The model under review builds one solid part; all positions refer to its coordinate system, in mm. Round coordinates to 2 decimals unless told otherwise and drop trailing zeros. Write each loop counter-clockwise with the first axis right and the second up, starting at its lowest first coordinate (ties: lowest second). Pieces come first, ordered by that corner, then holes.
Item 1: Add section C-C (z = -26). Give the boundary of the cut face in (x, y) (3 decimals).
Item 2: Add section A-A (x = 9). Give the boundary of the cut face in (y, z) (3 decimals), plus the area to 3 significant figures.
Item 3: Add section D-D (y = 1.1). State how many separate pieces and enclosed holes the cut face has, plus the area to 3 significant figures.
Item 4: Draft analysis for pull direction X (two halves, no side actions). For faces 1 (the face through (13, 2, -1.384)), 2 (the face through (29, 2, -33.274)), state which applies: +X half, -X half, draft (parallel to the pull), parting line (faces both ways), or undercut.
Item 5: Add section B-B (z = -31). Give the boundary of the cut face in (x, y) (3 decimals).
Item 6: Clearance check with flat-ended pins moving along their axes: pin 1 Ø1.5 at (y, z) = (2.5, -21) entering from -X; pin 2 Ø1 at (y, z) = (1, -4) entering from +X; pin 3 Ø4.5 at (x, z) = (52.57, -11.63) entering from -Y. State where each tip first meets the part, or that it passes through.
Item 7: To check wall thickness, follow L1, parallel to Z at x = 14, y = 1.3 (3 decimals); L2, parallel to X at y = 1.3, z = -11.5; L3, parallel to Z at x = 4, y = 1. State the ranges of each line that lie inside material, in increasing order.
```python
from build123d import *

# Parameters (mm, degrees)
BOSS_EXTRUDE1_DEPTH   = 3.175
F_6_32_TAPPED_HOLE1_D = 2.7051
CUT_EXTRUDE1_REACH    = 69.902


with BuildPart() as part:
    # Sketch1 → Boss-Extrude1 (new body)
    with BuildSketch(Plane(origin=(0, 0, 0), x_dir=(1, 0, 0), z_dir=(0, 1, 0))):
        with BuildLine():
            Line((3.175, 0), (53.721, 0))
            ThreePointArc((53.721, 0), (55.96606403, 0.92993597), (56.896, 3.175))
            Line((56.896, 3.175), (56.896, 11.684))
            ThreePointArc((56.896, 11.684), (59.1058, 16.637), (56.896, 21.59))
            Line((56.896, 21.59), (56.896, 30.099))
            ThreePointArc((56.896, 30.099), (55.96606403, 32.34406403), (53.721, 33.274))
            Line((53.721, 33.274), (3.175, 33.274))
            ThreePointArc((3.175, 33.274), (0.92993597, 32.34406403), (0, 30.099))
            Line((0, 30.099), (0, 21.59))
            ThreePointArc((0, 21.59), (-2.2098, 16.637), (0, 11.684))
            Line((0, 11.684), (0, 3.175))
            ThreePointArc((0, 3.175), (0.92993597, 0.92993597), (3.175, 0))
        make_face()
        with BuildLine():
            Line((49.276, 26.797), (7.62, 26.797))
            ThreePointArc((7.62, 26.797), (5.23875, 24.41575), (7.62, 22.0345))
            Line((7.62, 22.0345), (7.62, 19.01825))
            Line((7.62, 19.01825), (4.445875862, 19.01825))
            ThreePointArc((4.445875862, 19.01825), (2.064625862, 16.637), (4.445875862, 14.25575))
            Line((4.445875862, 14.25575), (7.62, 14.25575))
            Line((7.62, 14.25575), (7.62, 11.2395))
            ThreePointArc((7.62, 11.2395), (5.23875, 8.85825), (7.62, 6.477))
            Line((7.62, 6.477), (49.276, 6.477))
            ThreePointArc((49.276, 6.477), (51.65725, 8.85825), (49.276, 11.2395))
            Line((49.276, 11.2395), (49.276, 14.25575))
            Line((49.276, 14.25575), (52.450124138, 14.25575))
            ThreePointArc((52.450124138, 14.25575), (54.831374138, 16.637), (52.450124138, 19.01825))
            Line((52.450124138, 19.01825), (49.276, 19.01825))
            Line((49.276, 19.01825), (49.276, 22.0345))
            ThreePointArc((49.276, 22.0345), (51.65725, 24.41575), (49.276, 26.797))
        make_face(mode=Mode.SUBTRACT)
    extrude(amount=BOSS_EXTRUDE1_DEPTH)

    # #6-32 Tapped Hole1 (through all)
    with Locations(Plane(origin=(0, 3.175, 0), x_dir=(1, 0, 0), z_dir=(0, 1, 0))):
        with Locations((4.3307, 21.6408), (4.3307, 11.6332), (52.5653, 11.6332), (52.5653, 21.6408)):
            Hole(F_6_32_TAPPED_HOLE1_D / 2)

    # Sketch5 → Cut-Extrude1 (cut, up to next)
    with BuildSketch(Plane(origin=(0, 3.175, 0), x_dir=(1, 0, 0), z_dir=(0, 1, 0)), mode=Mode.PRIVATE) as cut_extrude1_sk1:
        with BuildLine():
            Line((23.9141, 31.8897), (25.0825, 31.8897))
            ThreePointArc((25.0825, 31.8897), (26.8605, 30.1117), (25.0825, 28.3337))
            Line((25.0825, 28.3337), (23.9141, 28.3337))
            ThreePointArc((23.9141, 28.3337), (22.1361, 30.1117), (23.9141, 31.8897))
        make_face()
    cut_extrude1_tool1 = extrude(cut_extrude1_sk1.sketch, amount=-CUT_EXTRUDE1_REACH, mode=Mode.PRIVATE) & part.part
    # Sketch5 → Cut-Extrude1 (cut, up to next)
    with BuildSketch(Plane(origin=(0, 3.175, 0), x_dir=(1, 0, 0), z_dir=(0, 1, 0)), mode=Mode.PRIVATE) as cut_extrude1_sk2:
        with BuildLine():
            Line((12.7635, 31.8897), (13.9319, 31.8897))
            ThreePointArc((13.9319, 31.8897), (15.7099, 30.1117), (13.9319, 28.3337))
            Line((13.9319, 28.3337), (12.7635, 28.3337))
            ThreePointArc((12.7635, 28.3337), (10.9855, 30.1117), (12.7635, 31.8897))
        make_face()
    cut_extrude1_tool2 = extrude(cut_extrude1_sk2.sketch, amount=-CUT_EXTRUDE1_REACH, mode=Mode.PRIVATE) & part.part
    # Sketch5 → Cut-Extrude1 (cut, up to next)
    with BuildSketch(Plane(origin=(0, 3.175, 0), x_dir=(1, 0, 0), z_dir=(0, 1, 0)), mode=Mode.PRIVATE) as cut_extrude1_sk3:
        with BuildLine():
            Line((4.8641, 31.8897), (6.0325, 31.8897))
            ThreePointArc((6.0325, 31.8897), (7.8105, 30.1117), (6.0325, 28.3337))
            Line((6.0325, 28.3337), (4.8641, 28.3337))
            ThreePointArc((4.8641, 28.3337), (3.0861, 30.1117), (4.8641, 31.8897))
        make_face()
    cut_extrude1_tool3 = extrude(cut_extrude1_sk3.sketch, amount=-CUT_EXTRUDE1_REACH, mode=Mode.PRIVATE) & part.part
    # Sketch5 → Cut-Extrude1 (cut, up to next)
    with BuildSketch(Plane(origin=(0, 3.175, 0), x_dir=(1, 0, 0), z_dir=(0, 1, 0)), mode=Mode.PRIVATE) as cut_extrude1_sk4:
        with BuildLine():
            Line((32.9819, 31.8897), (31.8135, 31.8897))
            ThreePointArc((31.8135, 31.8897), (30.0355, 30.1117), (31.8135, 28.3337))
            Line((31.8135, 28.3337), (32.9819, 28.3337))
            ThreePointArc((32.9819, 28.3337), (34.7599, 30.1117), (32.9819, 31.8897))
        make_face()
    cut_extrude1_tool4 = extrude(cut_extrude1_sk4.sketch, amount=-CUT_EXTRUDE1_REACH, mode=Mode.PRIVATE) & part.part
    # Sketch5 → Cut-Extrude1 (cut, up to next)
    with BuildSketch(Plane(origin=(0, 3.175, 0), x_dir=(1, 0, 0), z_dir=(0, 1, 0)), mode=Mode.PRIVATE) as cut_extrude1_sk5:
        with BuildLine():
            Line((44.1325, 31.8897), (42.9641, 31.8897))
            ThreePointArc((42.9641, 31.8897), (41.1861, 30.1117), (42.9641, 28.3337))
            Line((42.9641, 28.3337), (44.1325, 28.3337))
            ThreePointArc((44.1325, 28.3337), (45.9105, 30.1117), (44.1325, 31.8897))
        make_face()
    cut_extrude1_tool5 = extrude(cut_extrude1_sk5.sketch, amount=-CUT_EXTRUDE1_REACH, mode=Mode.PRIVATE) & part.part
    # Sketch5 → Cut-Extrude1 (cut, up to next)
    with BuildSketch(Plane(origin=(0, 3.175, 0), x_dir=(1, 0, 0), z_dir=(0, 1, 0)), mode=Mode.PRIVATE) as cut_extrude1_sk6:
        with BuildLine():
            Line((52.0319, 31.8897), (50.8635, 31.8897))
            ThreePointArc((50.8635, 31.8897), (49.0855, 30.1117), (50.8635, 28.3337))
            Line((50.8635, 28.3337), (52.0319, 28.3337))
            ThreePointArc((52.0319, 28.3337), (53.8099, 30.1117), (52.0319, 31.8897))
        make_face()
    cut_extrude1_tool6 = extrude(cut_extrude1_sk6.sketch, amount=-CUT_EXTRUDE1_REACH, mode=Mode.PRIVATE) & part.part
    # Sketch5 → Cut-Extrude1 (cut, up to next)
    with BuildSketch(Plane(origin=(0, 3.175, 0), x_dir=(1, 0, 0), z_dir=(0, 1, 0)), mode=Mode.PRIVATE) as cut_extrude1_sk7:
        with BuildLine():
            Line((52.0319, 1.3843), (50.8635, 1.3843))
            ThreePointArc((50.8635, 1.3843), (49.0855, 3.1623), (50.8635, 4.9403))
            Line((50.8635, 4.9403), (52.0319, 4.9403))
            ThreePointArc((52.0319, 4.9403), (53.8099, 3.1623), (52.0319, 1.3843))
        make_face()
    cut_extrude1_tool7 = extrude(cut_extrude1_sk7.sketch, amount=-CUT_EXTRUDE1_REACH, mode=Mode.PRIVATE) & part.part
    # Sketch5 → Cut-Extrude1 (cut, up to next)
    with BuildSketch(Plane(origin=(0, 3.175, 0), x_dir=(1, 0, 0), z_dir=(0, 1, 0)), mode=Mode.PRIVATE) as cut_extrude1_sk8:
        with BuildLine():
            Line((44.1325, 1.3843), (42.9641, 1.3843))
            ThreePointArc((42.9641, 1.3843), (41.1861, 3.1623), (42.9641, 4.9403))
            Line((42.9641, 4.9403), (44.1325, 4.9403))
            ThreePointArc((44.1325, 4.9403), (45.9105, 3.1623), (44.1325, 1.3843))
        make_face()
    cut_extrude1_tool8 = extrude(cut_extrude1_sk8.sketch, amount=-CUT_EXTRUDE1_REACH, mode=Mode.PRIVATE) & part.part
    # Sketch5 → Cut-Extrude1 (cut, up to next)
    with BuildSketch(Plane(origin=(0, 3.175, 0), x_dir=(1, 0, 0), z_dir=(0, 1, 0)), mode=Mode.PRIVATE) as cut_extrude1_sk9:
        with BuildLine():
            Line((32.9819, 1.3843), (31.8135, 1.3843))
            ThreePointArc((31.8135, 1.3843), (30.0355, 3.1623), (31.8135, 4.9403))
            Line((31.8135, 4.9403), (32.9819, 4.9403))
            ThreePointArc((32.9819, 4.9403), (34.7599, 3.1623), (32.9819, 1.3843))
        make_face()
    cut_extrude1_tool9 = extrude(cut_extrude1_sk9.sketch, amount=-CUT_EXTRUDE1_REACH, mode=Mode.PRIVATE) & part.part
    # Sketch5 → Cut-Extrude1 (cut, up to next)
    with BuildSketch(Plane(origin=(0, 3.175, 0), x_dir=(1, 0, 0), z_dir=(0, 1, 0)), mode=Mode.PRIVATE) as cut_extrude1_sk10:
        with BuildLine():
            Line((23.9141, 1.3843), (25.0825, 1.3843))
            ThreePointArc((25.0825, 1.3843), (26.8605, 3.1623), (25.0825, 4.9403))
            Line((25.0825, 4.9403), (23.9141, 4.9403))
            ThreePointArc((23.9141, 4.9403), (22.1361, 3.1623), (23.9141, 1.3843))
        make_face()
    cut_extrude1_tool10 = extrude(cut_extrude1_sk10.sketch, amount=-CUT_EXTRUDE1_REACH, mode=Mode.PRIVATE) & part.part
    # Sketch5 → Cut-Extrude1 (cut, up to next)
    with BuildSketch(Plane(origin=(0, 3.175, 0), x_dir=(1, 0, 0), z_dir=(0, 1, 0)), mode=Mode.PRIVATE) as cut_extrude1_sk11:
        with BuildLine():
            Line((12.7635, 1.3843), (13.9319, 1.3843))
            ThreePointArc((13.9319, 1.3843), (15.7099, 3.1623), (13.9319, 4.9403))
            Line((13.9319, 4.9403), (12.7635, 4.9403))
            ThreePointArc((12.7635, 4.9403), (10.9855, 3.1623), (12.7635, 1.3843))
        make_face()
    cut_extrude1_tool11 = extrude(cut_extrude1_sk11.sketch, amount=-CUT_EXTRUDE1_REACH, mode=Mode.PRIVATE) & part.part
    # Sketch5 → Cut-Extrude1 (cut, up to next)
    with BuildSketch(Plane(origin=(0, 3.175, 0), x_dir=(1, 0, 0), z_dir=(0, 1, 0)), mode=Mode.PRIVATE) as cut_extrude1_sk12:
        with BuildLine():
            Line((4.8641, 1.3843), (6.0325, 1.3843))
            ThreePointArc((6.0325, 1.3843), (7.8105, 3.1623), (6.0325, 4.9403))
            Line((6.0325, 4.9403), (4.8641, 4.9403))
            ThreePointArc((4.8641, 4.9403), (3.0861, 3.1623), (4.8641, 1.3843))
        make_face()
    cut_extrude1_tool12 = extrude(cut_extrude1_sk12.sketch, amount=-CUT_EXTRUDE1_REACH, mode=Mode.PRIVATE) & part.part
    add(cut_extrude1_tool1.solids().sort_by_distance((24.4983, 3.175, -30.1117))[0], mode=Mode.SUBTRACT)
    add(cut_extrude1_tool2.solids().sort_by_distance((13.3477, 3.175, -30.1117))[0], mode=Mode.SUBTRACT)
    add(cut_extrude1_tool3.solids().sort_by_distance((5.4483, 3.175, -30.1117))[0], mode=Mode.SUBTRACT)
    add(cut_extrude1_tool4.solids().sort_by_distance((32.3977, 3.175, -30.1117))[0], mode=Mode.SUBTRACT)
    add(cut_extrude1_tool5.solids().sort_by_distance((43.5483, 3.175, -30.1117))[0], mode=Mode.SUBTRACT)
    add(cut_extrude1_tool6.solids().sort_by_distance((51.4477, 3.175, -30.1117))[0], mode=Mode.SUBTRACT)
    add(cut_extrude1_tool7.solids().sort_by_distance((51.4477, 3.175, -3.1623))[0], mode=Mode.SUBTRACT)
    add(cut_extrude1_tool8.solids().sort_by_distance((43.5483, 3.175, -3.1623))[0], mode=Mode.SUBTRACT)
    add(cut_extrude1_tool9.solids().sort_by_distance((32.3977, 3.175, -3.1623))[0], mode=Mode.SUBTRACT)
    add(cut_extrude1_tool10.solids().sort_by_distance((24.4983, 3.175, -3.1623))[0], mode=Mode.SUBTRACT)
    add(cut_extrude1_tool11.solids().sort_by_distance((13.3477, 3.175, -3.1623))[0], mode=Mode.SUBTRACT)
    add(cut_extrude1_tool12.solids().sort_by_distance((5.4483, 3.175, -3.1623))[0], mode=Mode.SUBTRACT)


solid = part.part
```
Numbers:
1. outline: (0, 0) - (5.842, 0) - (5.842, 3.175) - (0, 3.175) - close; (51.054, 0) - (56.896, 0) - (56.896, 3.175) - (51.054, 3.175) - close
2. outline: (0, -33.274) - (3.175, -33.274) - (3.175, -26.797) - (0, -26.797) - close; (0, -6.477) - (3.175, -6.477) - (3.175, 0) - (0, 0) - close
2. area: 41.1 mm2
3. separate pieces: 1
3. enclosed holes: 17
3. area: 793 mm2
4. face 1: undercut
4. face 2: draft
5. outline: (0.131, 0) - (3.324, 0) - (3.324, 3.175) - (0.131, 3.175) - close; (7.573, 0) - (11.223, 0) - (11.223, 3.175) - (7.573, 3.175) - close; (15.472, 0) - (22.374, 0) - (22.374, 3.175) - (15.472, 3.175) - close; (26.623, 0) - (30.273, 0) - (30.273, 3.175) - (26.623, 3.175) - close; (34.522, 0) - (41.424, 0) - (41.424, 3.175) - (34.522, 3.175) - close; (45.673, 0) - (49.323, 0) - (49.323, 3.175) - (45.673, 3.175) - close; (53.572, 0) - (56.765, 0) - (56.765, 3.175) - (53.572, 3.175) - close
6. pin 1: stops at x = -1.14
6. pin 2: stops at x = 56.9
6. pin 3: stops at y = 0
7. L1: z = -33.274 to -31.888, -28.335 to -26.797, -6.477 to -4.939, -1.386 to 0
7. L2: x = 0 to 2.98, 5.68 to 7.62, 49.28 to 51.22, 53.91 to 56.9
7. L3: z = -33.27 to -31.67, -28.56 to -22.95, -20.33 to -18.98, -14.3 to -12.94, -10.32 to -4.72, -1.61 to 0
